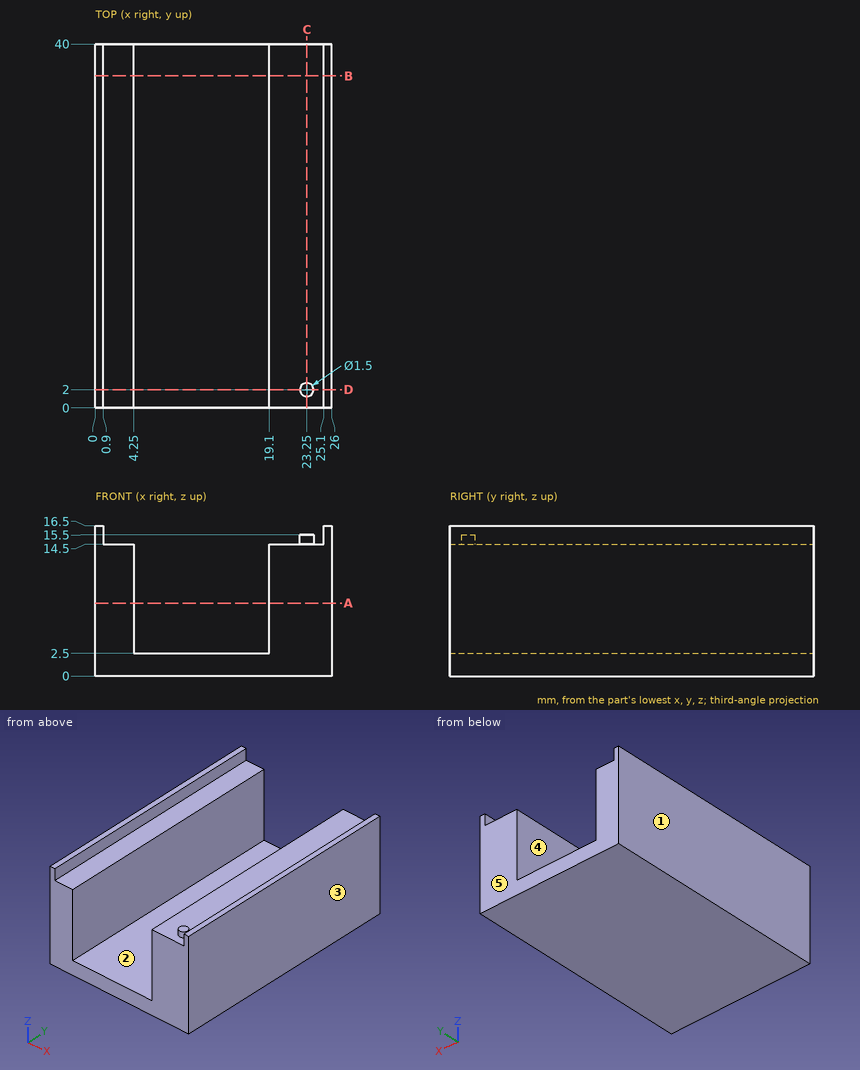
Can you work these out from the drawing? Everything is in mm from the part's minimum corner. A direction names the side the tool comes from. Round coordinates to 2 decimals unless told otherwise and drop trailing zeros. Loops run counter-clockwise (first coordinate to the right, second up) from the corner with the lowest first, then second, coordinate; pieces in that order, holes last.
1. If we section it at D-D on y = 2: Write out the boundary of the cut face in (x, z), plus the area to 3 significant figures.
Answer list:
outline: (0, 0) - (26, 0) - (26, 16.5) - (25.1, 16.5) - (25.1, 14.5) - (24, 14.5) - (24, 15.5) - (22.5, 15.5) - (22.5, 14.5) - (19.1, 14.5) - (19.1, 2.5) - (4.25, 2.5) - (4.25, 14.5) - (0.9, 14.5) - (0.9, 16.5) - (0, 16.5) - close
area: 204 mm2
2. Which directions (+Z, -Z, +X, -X, +Y, -Y) give clear straight access to the entire face, cutting with the end or side of a thin tool? Please do the marked faces 4 and 5.
Answer list:
face 4: +Z, +Y, -Y
face 5: +Z, -Z, +X, -X, +Y
3. If I drill on line 1 along X through (y, z) = (16, 10.5); line 2 along X through (y, z) = (7, 15.25); line 3 along Z through (x, y) = (10.5, 33), over which ranges is the centre line in solid material (lowest first)?
Answer list:
line 1: x = 0 to 4.25, 19.1 to 26
line 2: x = 0 to 0.9, 25.1 to 26
line 3: z = 0 to 2.5
4. If we section it at B-B on y = 36.5: Write out the boundary of the cut face in (x, z).
Answer list:
outline: (0, 0) - (26, 0) - (26, 16.5) - (25.1, 16.5) - (25.1, 14.5) - (19.1, 14.5) - (19.1, 2.5) - (4.25, 2.5) - (4.25, 14.5) - (0.9, 14.5) - (0.9, 16.5) - (0, 16.5) - close
5. If we section it at A-A on z = 8: Write out the boundary of the cut face in (x, y).
Answer list:
outline: (0, 0) - (4.25, 0) - (4.25, 40) - (0, 40) - close; (19.1, 0) - (26, 0) - (26, 40) - (19.1, 40) - close
6. For P1, Ø0.8, axis at x = 23.5, y = 2, coming from the +Z side; P2, Ø1, axis at x = 17, y = 25, coming from the +Z side; P3, Ø2.5, axis at x = 2.5, y = 21.5, coming from the +Z side, each with a flat end and sliding along its axis, tell me the tip position at first contact or that it passes through.
Answer list:
P1: stops at z = 15.5
P2: stops at z = 2.5
P3: stops at z = 14.5
7. We'd pull the mould along X, two halves only. Please class the marked faces 1, 2 and 3: +X half, -X half, draft (parallel to the pull), parting line (faces both ways), or undercut.
Answer list:
face 1: -X half
face 2: undercut
face 3: +X half
8. If we section it at C-C on x = 23.25: Write out the boundary of the cut face in (y, z), plus the area to 4 significant figures.
Answer list:
outline: (0, 0) - (40, 0) - (40, 14.5) - (2.75, 14.5) - (2.75, 15.5) - (1.25, 15.5) - (1.25, 14.5) - (0, 14.5) - close
area: 581.5 mm2
